Work out the finished part from the listing and answer in its coordinate system (mm). Face numbers are marked on the shaded views. A direction names the side the tool comes from. Round coordinates to 2 decimals unless told otherwise and drop trailing zeros. Order: outer loops, then holes, each group sorted by start corner. A loop starts at its lowest first (then second) coordinate and runs counter-clockwise, first axis right, second up. Notation, with made-up numbers: M -3.5,-32.75 L 42.5,-32.75 A27 ccw 42.5,-14.75 Z; hole C 25.25,-35.5 d11. An arc over 180 degrees is marked long. Return JSON: item names as keys, results as strings.
from build123d import *

# Parameters (mm, degrees)
SKETCH1_W           = 762
SKETCH1_H           = 203.2
BOSS_EXTRUDE1_DEPTH = 76.2
SKETCH2_W           = 203.2
SKETCH2_H           = 95.25
CUT_EXTRUDE1_DEPTH  = 63.5
SKETCH3_W           = 203.2
SKETCH3_H           = 38.1
CUT_EXTRUDE2_DEPTH  = 792.18044086
FILLET1_R           = 25.4


with BuildPart() as part:
    # Sketch1 → Boss-Extrude1 (new body)
    with BuildSketch(Plane(origin=(0, 0, 0), x_dir=(0, 0, -1), z_dir=(1, 0, 0))):
        with Locations((381, 101.6)):
            Rectangle(SKETCH1_W, SKETCH1_H)
    extrude(amount=BOSS_EXTRUDE1_DEPTH)

    # Sketch2 → Cut-Extrude1 (cut)
    with BuildSketch(Plane.ZY):
        with Locations((-381, 92.075)):
            Rectangle(SKETCH2_W, SKETCH2_H)
    extrude(amount=-CUT_EXTRUDE1_DEPTH, mode=Mode.SUBTRACT)

    # Sketch3 → Cut-Extrude2 (cut, through all)
    with BuildSketch(Plane.ZY.offset(-63.5)):
        with Locations((-381, 76.2)):
            Rectangle(SKETCH3_W, SKETCH3_H)
    extrude(amount=-CUT_EXTRUDE2_DEPTH, mode=Mode.SUBTRACT)

    # Fillet1
    fillet1_edges = [part.edges().sort_by_distance(p)[0] for p in [
        (31.75, 139.7, -482.6),
        (31.75, 139.7, -279.4),
    ]]
    fillet(fillet1_edges, radius=FILLET1_R)


solid = part.part
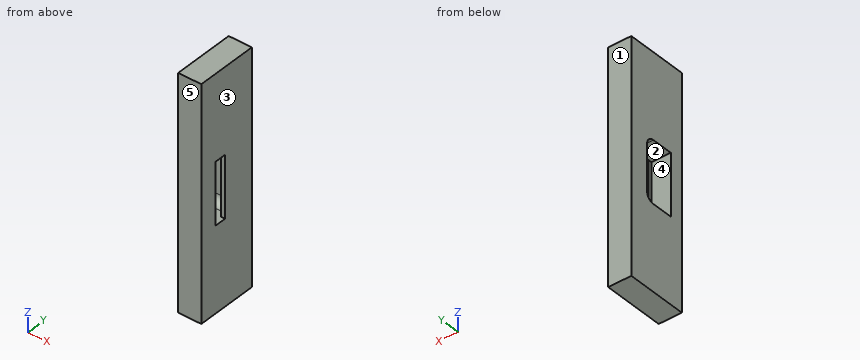
Item 1: Find section A-A (z = -434.5). Determine the outline of the cut face in (x, y), plus the area to 3 significant figures.
Output:
{"outline": "M 0,0 L 76.2,0 L 76.2,57.15 L 63.5,57.15 L 63.5,44.45 L 0,44.45 Z; M 0,139.7 L 63.5,139.7 L 63.5,95.25 L 76.2,95.25 L 76.2,203.2 L 0,203.2 Z", "area": "8,950 mm^2"}
Item 2: Which of the six approach directions +Z, -Z, +X, -X, +Y, -Y give full straight-line access (tool end or side, diameter ignored) to the marked faces 1 and 2?
Output:
{"face 1": "+Z, -Z, +X, -X, +Y", "face 2": "-X"}
Item 3: The mould has two halves that part along Y. Classify the marked faces 3, 4 and 5: pulls with the +Y half, pulls with the -Y half, needs draft (parallel to the pull), parting line crosses it, or undercut.
Output:
{"face 3": "needs draft", "face 4": "undercut", "face 5": "pulls with the -Y half"}
Item 4: Consider line 1 along Z through (x, y) = (53.5, 71); line 2 along Y through (x, z) = (7.5, -346.5); line 3 along X through (y, z) = (125.5, -306.5). Determine where each line is inside the solid, lowest interval first. Write a range as [from, to].
Output:
{"line 1": "z = [-762, -482.6], [-279.4, 0]", "line 2": "y = [0, 44.45], [139.7, 203.2]", "line 3": "x = [63.5, 76.2]"}
Item 5: Find section C-C (x = 50). Determine the outline of the cut face in (y, z), plus the area to 3 significant figures.
Output:
{"outline": "M 0,-762 L 203.2,-762 L 203.2,0 L 0,0 Z; hole M 44.45,-482.6 L 114.3,-482.6 A25.4 ccw 139.7,-457.2 L 139.7,-304.8 A25.4 ccw 114.3,-279.4 L 44.45,-279.4 Z", "area": "136,000 mm^2"}
Item 6: This flat-tipped pin is pushed along its axis until it touches: pin 1 (6.5 mm diameter, centred on y = 48.5, z = -406, fed in from -X). Where does it stop, or does it pass through?
Output:
{"pin 1": "stops at x = 63.5"}
Item 7: Find section B-B (y = 66). Determine the outline of the cut face in (x, z), plus the area to 3 significant figures.
Output:
{"outline": "M 0,-762 L 76.2,-762 L 76.2,-482.6 L 0,-482.6 Z; M 0,-279.4 L 76.2,-279.4 L 76.2,0 L 0,0 Z", "area": "42,600 mm^2"}
